```python
from build123d import *

# Parameters (mm, degrees)
F0_W     = 180
F0_H     = 125
F1_DEPTH = 10
F3_DEPTH = 5
F4_W     = 76
F4_H     = 28.5
F5_DEPTH = 5.001


with BuildPart() as f1:
    # F0 (on Top) → F1 (new body)
    with BuildSketch(Plane.XY):
        Rectangle(F0_W, F0_H)
    extrude(amount=F1_DEPTH)

    # F2 (on face) → F3 (cut)
    with BuildSketch(Plane(origin=(0, 0, 0), x_dir=(1, 0, 0), z_dir=(0, 0, -1))):
        with BuildLine():
            Line((70, 12.5), (70, 37.5))
            ThreePointArc((70, 37.5), (68.535534, 41.035534), (65, 42.5))
            Line((65, 42.5), (-15, 42.5))
            ThreePointArc((-15, 42.5), (-18.535534, 41.035534), (-20, 37.5))
            Line((-20, 37.5), (-20, 12.5))
            ThreePointArc((-20, 12.5), (-18.535534, 8.964466), (-15, 7.5))
            Line((-15, 7.5), (65, 7.5))
            ThreePointArc((65, 7.5), (68.535534, 8.964466), (70, 12.5))
        make_face()
    extrude(amount=-F3_DEPTH, mode=Mode.SUBTRACT)

    # F4 (on face) → F5 (cut, through all)
    with BuildSketch(Plane(origin=(0, 0, 5), x_dir=(1, 0, 0), z_dir=(0, 0, -1))):
        with Locations((25, 21.75)):
            Rectangle(F4_W, F4_H)
    extrude(amount=-F5_DEPTH, mode=Mode.SUBTRACT)


solid = f1.part
```
Can you work these out from the model? Positions are in its coordinate system, mm. A direction names the side the tool comes from. Give positions to 0.01 mm unless a question says otherwise; leave off trailing zeros. Order: outer loops, then holes, each group sorted by start corner. A loop starts at its lowest first (then second) coordinate and runs counter-clockwise, first axis right, second up. Notation, with made-up numbers: (19, 50.5) - (42, 50.5) arc R31 ccw to (42, 88.5) - close; hole circle Ø2 at (88.5, -10). An arc over 180 degrees is marked (long way). Use a Markdown table: item, result. Add a question column.
Q1. Please list where these lines run through material, in increasing order: line 1 along X through (y, z) = (-17, 8.25); line 2 along Y through (x, z) = (-5.5, 7.75); line 3 along Y through (x, z) = (-11, 3.25).
Q2. On a 3-axis mill with a long thin cutter (end or side, diameter ignored), from which of +Z, -Z, +X, -X, +Y, -Y can I reach the whole of each face in a straight line? I mean faces 5 (the cylindrical face through (68.5, -8.93, 2.46)), 6 (the flat face through (24, -36, 7)), 7 (the flat face through (-90, -1, 5)). Say none if no direction works.
Q3. If we section it at A-A on x = 2: Write out the boundary of the cut face in (y, z).
Q4. If we section it at B-B on z = 3.25: Write out the boundary of the cut face in (x, y), plus the area to 3 significant figures.
Q5. I'm going to push a flat-ended pin straight in: pin 1 (10.5 mm diameter, centred on x = 26.5, y = -31.5, fed in from -Z). Where does the tip first touch, or does it pass through?
Q6. If we mould it in two halves opening along Y, with no side actions, what happens to faces 1 (the flat face through (-1, 62.5, 5)), 2 (the flat face through (90, -1, 5)), 3 (the flat face through (24, -37, 5)), 4 (the flat face through (-1, -62.5, 5))? For each: released by +Y, released by -Y, zero draft, split by the parting line, or undercut.
Answers follow:
| question | item | result |
|---|---|---|
| 1 | line 1 | x = -90 to -13, 63 to 90 |
| 1 | line 2 | y = -62.5 to -36, -7.5 to 62.5 |
| 1 | line 3 | y = -62.5 to -42.5, -7.5 to 62.5 |
| 2 | face 5 | -Z |
| 2 | face 6 | +Z, -Z |
| 2 | face 7 | +Z, -Z, -X, +Y, -Y |
| 3 | outline | (-62.5, 0) - (-42.5, 0) - (-42.5, 5) - (-36, 5) - (-36, 10) - (-62.5, 10) - close; (-7.5, 0) - (62.5, 0) - (62.5, 10) - (-7.5, 10) - close |
| 4 | outline | (-90, -62.5) - (90, -62.5) - (90, 62.5) - (-90, 62.5) - close; hole (-20, -37.5) arc R5 ccw to (-15, -42.5) - (65, -42.5) arc R5 ccw to (70, -37.5) - (70, -12.5) arc R5 ccw to (65, -7.5) - (-15, -7.5) arc R5 ccw to (-20, -12.5) - close |
| 4 | area | 19,400 mm^2 |
| 5 | pin 1 | stops at z = 5 |
| 6 | face 1 | released by +Y |
| 6 | face 2 | zero draft |
| 6 | face 3 | undercut |
| 6 | face 4 | released by -Y |
